The figure shows three views and two pictorial views of one solid part (mm, origin at its lowest corner). Answer the questions. Give positions to 0.01 mm unless a question says otherwise; leave off trailing zeros. Loops run counter-clockwise (first coordinate to the right, second up) from the corner with the lowest first, then second, coordinate; pieces in that order, holes last. Notation, with made-up numbers: (-29.5, -24.75) - (14.5, -24.75) arc R19 ccw to (14.5, 8.25) - close; hole circle Ø2 at (80, -10). An arc over 180 degrees is marked (long way). One line per question, with ' | ' between items.
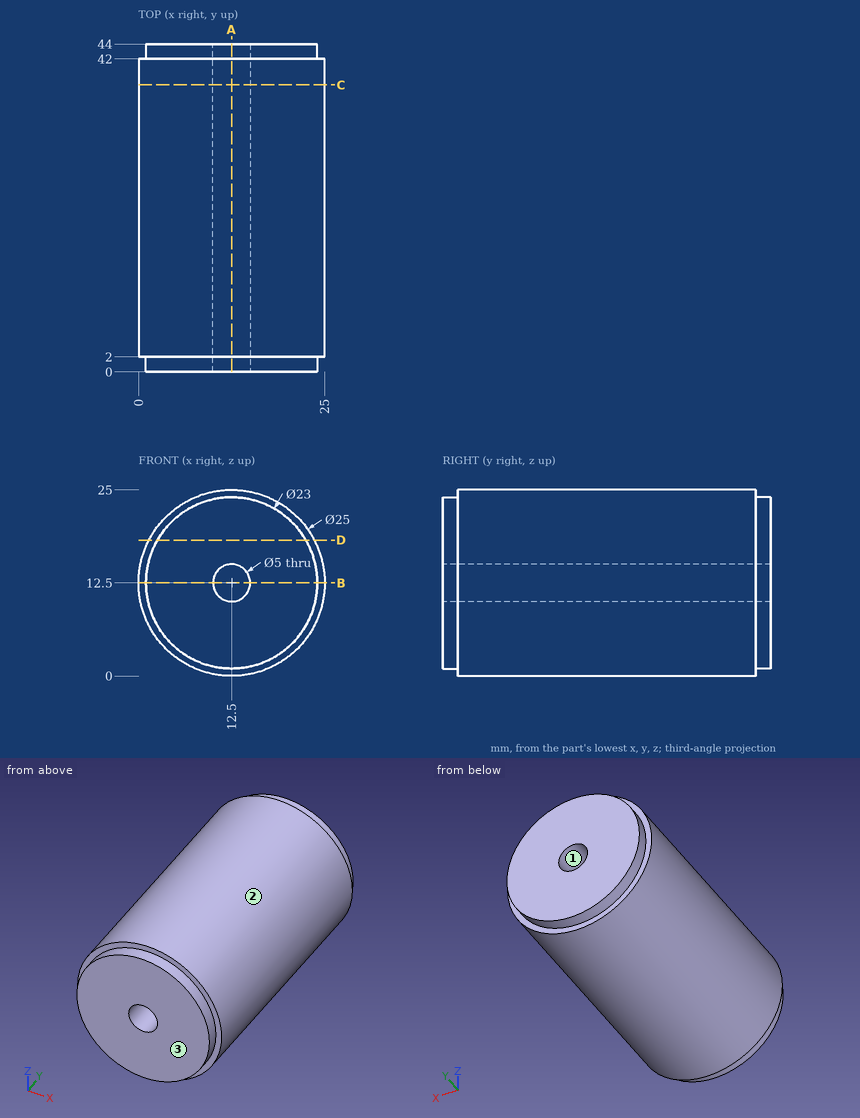
1. Determine the mould class of the marked faces 1, 2 and 3 for opening direction X: +X half, -X half, draft (parallel to the pull), parting line (faces both ways), or undercut.
Evaluation:
face 1: undercut | face 2: parting line | face 3: draft
2. Find section A-A on x = 12.5. Write down the section's boundary in (y, z).
Evaluation:
outline: (0, 1) - (2, 1) - (2, 0) - (42, 0) - (42, 1) - (44, 1) - (44, 10) - (0, 10) - close; (0, 15) - (44, 15) - (44, 24) - (42, 24) - (42, 25) - (2, 25) - (2, 24) - (0, 24) - close
3. Find section B-B on z = 12.5. Write down the section's boundary in (x, y), then the cut area to 3 significant figures.
Evaluation:
outline: (0, 2) - (1, 2) - (1, 0) - (10, 0) - (10, 44) - (1, 44) - (1, 42) - (0, 42) - close; (15, 0) - (24, 0) - (24, 2) - (25, 2) - (25, 42) - (24, 42) - (24, 44) - (15, 44) - close | area: 872 mm2
4. Find section D-D on z = 18.25. Write down the section's boundary in (x, y), then the cut area to 3 significant figures.
Evaluation:
outline: (1.4, 2) - (2.54, 2) - (2.54, 0) - (22.46, 0) - (22.46, 2) - (23.6, 2) - (23.6, 42) - (22.46, 42) - (22.46, 44) - (2.54, 44) - (2.54, 42) - (1.4, 42) - close | area: 968 mm2
5. Find section C-C on y = 38.5. Write down the section's boundary in (x, z), then the cut area to 3 significant figures.
Evaluation:
outline: circle Ø25 at (12.5, 12.5); hole circle Ø5 at (12.5, 12.5) | area: 471 mm2
6. Flat-ended cylindrical pins translate along their axes: pin 1 (2 mm diameter, centred on x = 3.5, y = 17.5, fed in from +Z); pin 2 (10 mm diameter, centred on x = 20.5, y = 14.5, fed in from -Z); pin 3 (6 mm diameter, centred on x = 16.5, y = 34, fed in from +Z). Find the tip coordinate at first contact, or state that the pin passes through.
Evaluation:
pin 1: z = 22.1 | pin 2: z = 0.37 | pin 3: z = 24.96
7. Consider L1, parallel to Z at x = 12.5, y = 34.5; L2, parallel to Z at x = 10.5, y = 16.5. Determine where each line is inside the solid, lowest interval first.
Evaluation:
L1: 0 to 10, 15 to 25 | L2: 0.16 to 11, 14 to 24.84
